Part model, mm, in its own coordinate system. Face numbers are marked on the shaded views. A direction names the side the tool comes from. Give positions to 0.01 mm unless a question says otherwise; leave off trailing zeros. Write each loop counter-clockwise with the first axis right and the second up, starting at its lowest first coordinate (ties: lowest second). Pieces come first, ordered by that corner, then holes. Notation, with made-up numbers: (59, 25.5) - (104, 25.5) arc R7 cw to (104, 32.5) - close; hole circle Ø3 at (34, -25.75). An arc over 180 degrees is marked (long way). Answer in a Markdown table with one row per item. Add a question column.
1. Band-saw the part on C-C on y = 17.5. Write the cut outline in (x, z).
2. Probe line 1 along Z through (x, y) = (46.5, 15.5); line 2 along Z through (x, y) = (59.5, 11.5); line 3 along Y through (x, z) = (11.5, 7.5). List the from-to ranges inside material, lowest first.
3. Drop flat-ended pins along their axis: pin 1 Ø3 at (x, z) = (18, 6) entering from -Y; pin 2 Ø4 at (x, z) = (50, -3) entering from -Y. Give the stop position or say it passes through.
4. Which spindle directions (+Z, -Z, +X, -X, +Y, -Y) get a long thin tool onto all of the face, cutting with end or side? Do the marked faces 1 and 2. Say none if no direction does.
5. Band-saw the part on D-D on z = -5.5. Write the cut outline in (x, y), plus the area to 3 significant figures.
6. Band-saw the part on A-A on y = 13. Write the cut outline in (x, z).
7. Band-saw the part on B-B on x = 47.5. Write the cut outline in (y, z).
```python
from build123d import *

# Parameters (mm, degrees)
SKETCH_1_W          = 56
SKETCH_1_H          = 56
EXTRUDE_1_DEPTH     = 36
SKETCH_3_R          = 12.893800992
CUT_EXTRUDE_5_DEPTH = 56
CUT_EXTRUDE_6_DEPTH = 56


with BuildPart() as part:
    # 草图1 → 凸台-拉伸1 (new body)
    with BuildSketch(Plane(origin=(0, 0, 0), x_dir=(1, 0, 0), z_dir=(0, 1, 0))):
        with Locations((36.119558337, -6.81415619)):
            Rectangle(SKETCH_1_W, SKETCH_1_H)
    extrude(amount=EXTRUDE_1_DEPTH)

    # 草图3 → 切除-拉伸5 (cut)
    with BuildSketch(Plane(origin=(64.119558337, 0, 0), x_dir=(0, 0, -1), z_dir=(1, 0, 0))):
        with Locations((-5.712666973, 16)):
            Circle(SKETCH_3_R)
        with BuildLine():
            ThreePointArc((7.181134019, 16), (-5.712666973, 3.106199008), (-18.606467966, 16))
            Line((-18.606467966, 16), (-18.606467966, 0))
            Line((-18.606467966, 0), (7.181134019, 0))
            Line((7.181134019, 0), (7.181134019, 16))
        make_face()
    extrude(amount=-CUT_EXTRUDE_5_DEPTH, mode=Mode.SUBTRACT)

    # 草图5 → 切除-拉伸6 (cut)
    with BuildSketch(Plane(origin=(0, 36, 0), x_dir=(1, 0, 0), z_dir=(0, 1, 0))):
        with BuildLine():
            ThreePointArc((54.119558337, -34.81415619), (64.119558337, -44.81415619), (74.119558337, -34.81415619))
            ThreePointArc((74.119558337, -34.81415619), (71.190626149, -27.743088379), (64.119558337, -24.81415619))
            Line((64.119558337, -24.81415619), (64.119558337, -34.81415619))
            Line((64.119558337, -34.81415619), (54.119558337, -34.81415619))
        make_face()
        with BuildLine():
            Line((64.119558337, -34.81415619), (64.119558337, -24.81415619))
            ThreePointArc((64.119558337, -24.81415619), (57.048490525, -27.743088379), (54.119558337, -34.81415619))
            Line((54.119558337, -34.81415619), (64.119558337, -34.81415619))
        make_face()
        with BuildLine():
            Line((8.119558337, 21.18584381), (18.119558337, 21.18584381))
            ThreePointArc((18.119558337, 21.18584381), (1.048490525, 28.256911621), (8.119558337, 11.18584381))
            Line((8.119558337, 11.18584381), (8.119558337, 21.18584381))
        make_face()
        with BuildLine():
            ThreePointArc((8.119558337, 11.18584381), (15.190626149, 14.114775998), (18.119558337, 21.18584381))
            Line((18.119558337, 21.18584381), (8.119558337, 21.18584381))
            Line((8.119558337, 21.18584381), (8.119558337, 11.18584381))
        make_face()
    extrude(amount=-CUT_EXTRUDE_6_DEPTH, mode=Mode.SUBTRACT)


solid = part.part
```
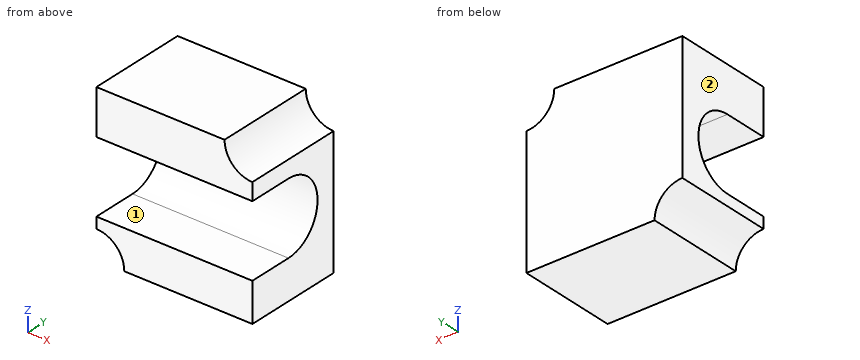
Values:
| question | item | result |
|---|---|---|
| 1 | outline | (8.12, -11.19) arc R10 cw to (18.12, -21.19) - (64.12, -21.19) - (64.12, -7.09) - (8.12, -7.09) - close; (8.12, 18.52) - (64.12, 18.52) - (64.12, 24.81) arc R10 cw to (54.12, 34.81) - (8.12, 34.81) - close |
| 2 | line 1 | z = -21.19 to -7.18, 18.61 to 34.81 |
| 2 | line 2 | z = -21.19 to -7.18, 18.61 to 25.95 |
| 2 | line 3 | y = 28.77 to 36 |
| 3 | pin 1 | stops at y = 28.77 |
| 3 | pin 2 | stops at y = 23.18 |
| 4 | face 1 | +X, -X, -Y |
| 4 | face 2 | +Z, -Z, -X, +Y, -Y |
| 5 | outline | (8.12, 22.37) - (64.12, 22.37) - (64.12, 36) - (8.12, 36) - close |
| 5 | area | 764 mm² |
| 6 | outline | (8.12, -11.19) arc R10 cw to (18.12, -21.19) - (64.12, -21.19) - (64.12, -7.18) - (8.12, -7.18) - close; (8.12, 18.61) - (64.12, 18.61) - (64.12, 24.81) arc R10 cw to (54.12, 34.81) - (8.12, 34.81) - close |
| 7 | outline | (0, -21.19) - (36, -21.19) - (36, 34.81) - (0, 34.81) - (0, 18.61) - (16, 18.61) arc R12.89 cw to (16, -7.18) - (0, -7.18) - close |
